```python
from build123d import *

# Parameters (mm, degrees)
F1_ANGLE = 180
F3_D     = 76.2
F4_R     = 165.2325510481
F5_DEPTH = 543.62825
F6_DEPTH = 601.10694


with BuildPart() as f1:
    # F0 (on Top) → F1 (revolve)
    with BuildSketch(Plane.XY):
        with BuildLine():
            Line((0, -444.5), (0, -457.2))
            ThreePointArc((0, -457.2), (457.2, 0), (0, 457.2))
            Line((0, 457.2), (0, 444.5))
            ThreePointArc((0, 444.5), (444.5, 0), (0, -444.5))
        make_face()
    revolve(axis=Axis((0, 0, 0), (0, -1, 0)), revolution_arc=F1_ANGLE)

    # F3 (through all)
    with Locations(Plane(origin=(0, 0, 0), x_dir=(1, 0, 0), z_dir=(0, 0, -1))):
        with Locations((-116.6023164988, 18.9869366586), (129.3481886387, -195.9198415279), (215.2733206749, 124.0054294467)):
            Hole(F3_D / 2)

    # F4 (on Top) → F5 (join)
    with BuildSketch(Plane.XY):
        with Locations((215.2733206749, -124.0054294467)):
            Circle(F4_R)
    extrude(amount=F5_DEPTH)

    # F6 (add): a face of the model
    f6_faces = [f1.faces().sort_by_distance(p)[0] for p in [
        (445.7931568814, 0, 0),
    ]]
    extrude(f6_faces, amount=F6_DEPTH)


solid = f1.part
```
Geometry: final body of the model. Coordinates: model frame, mm. A direction names the side the tool comes from. Coordinates: 2 decimals unless noted, no trailing zeros. Order: outer loops, then holes, each group sorted by start corner. A loop starts at its lowest first (then second) coordinate and runs counter-clockwise, first axis right, second up. Notation, with made-up numbers: M -23,1.25 L 15,1.25 A35 ccw 15,39.25 Z; hole C 64.25,7 d2. An arc over 180 degrees is marked long. Answer as CSV lines item,"result".
Q1. Section A-A on y = 0. Return the cut outline in (x, z), and give its area (3 significant figures).
Answers:
outline,"M -457.2,-601.11 L -444.5,-601.11 L -444.5,0 A444.5 cw -149.63,418.56 L -149.63,432.02 A457.2 ccw -457.2,0 Z; M -83.57,436.57 A444.5 cw 106.07,431.66 L 106.07,0 L 324.47,0 L 324.47,303.81 A444.5 cw 444.5,0 L 444.5,-601.11 L 457.2,-601.11 L 457.2,0 A457.2 ccw 324.47,322.1 L 324.47,543.63 L 106.07,543.63 L 106.07,444.72 A457.2 ccw -83.57,449.5 Z"
area,"148,000 mm^2"
Q2. First-contact query: P1, Ø12, axis at x = -226, z = -428.5, coming from the +Y side; P2, Ø4, axis at y = -193, z = -50, coming from the -X side; P3, Ø8, axis at x = -357, y = -65.5, coming from the +Z side. Flat tips, straight axial feed; report the tip coordinate or a pass-through.
Answers:
P1,"stops at y = 400.79"
P2,"stops at x = -415.39"
P3,"stops at z = 283.16"
Q3. Line query: probe 1 along X at (y, z) = (0, -341); probe 2 along X at (y, z) = (-73, 31.5); probe 3 along X at (y, z) = (217, -365). Output: solid intervals per line, ascending. Write a range as [from, to].
Answers:
probe 1,"x = [-457.2, -444.5], [444.5, 457.2]"
probe 2,"x = [-450.23, -437.33], [58.11, 372.44], [437.33, 450.23]"
probe 3,"x = [-402.42, -387.93], [387.93, 402.42]"
Q4. Section B-B on x = 140. Return the cut outline in (y, z), and give its area (3 significant figures).
Answers:
outline,"M -435.24,-601.11 L -421.88,-601.11 L -421.88,0 A421.88 cw -271.1,323.24 L -271.1,0 L 23.09,0 L 23.09,421.24 A421.88 cw 159.34,390.63 L 159.34,405.02 A435.24 ccw 23.09,434.63 L 23.09,543.63 L -271.1,543.63 L -271.1,340.5 A435.24 ccw -435.24,0 Z; M 232.5,352.03 A421.88 cw 421.88,0 L 421.88,-601.11 L 435.24,-601.11 L 435.24,0 A435.24 ccw 232.5,367.93 Z"
area,"189,000 mm^2"
Q5. Set-up query: faces 1 (the cylindrical face through (103.6, 224, 382)), 2 (the cylindrical face through (367.906, -187.29, 405.492)), 3 (the flat face through (213, -122, 0)). Return all of +Z, -Z, +X, -X, +Y, -Y with unobstructed straight access to the full face (end or side cutting, diameter ignored); none if empty.
Answers:
face 1,"+Z, -Z"
face 2,"+Z"
face 3,"-Z"
Q6. Section D-D on y = -148. Return the cut outline in (x, z), and give its area (3 significant figures).
Answers:
outline,"M -432.58,-601.11 L -419.14,-601.11 L -419.14,0 A419.14 cw 51.79,415.93 L 51.79,0 L 378.75,0 L 378.75,179.5 A419.14 cw 419.14,0 L 419.14,-601.11 L 432.58,-601.11 L 432.58,0 A432.58 ccw 378.75,208.98 L 378.75,543.63 L 51.79,543.63 L 51.79,429.47 A432.58 ccw -432.58,0 Z"
area,"206,000 mm^2"
Q7. Section C-C on z = 99.5. Return the cut outline in (x, y), and give its area (3 significant figures).
Answers:
outline,"C 0,0 d892.48; C 215.27,-124.01 d330.47; hole C 0,0 d866.44"
area,"122,000 mm^2"
